Read the model definition and answer for the solid it produces. Units are mm, in the model's axes. A direction names the side the tool comes from. Coordinates: 2 decimals unless noted, no trailing zeros. Loops run counter-clockwise (first coordinate to the right, second up) from the corner with the lowest first, then second, coordinate; pieces in that order, holes last. Notation, with made-up numbers: (67, 78.25) -> (84, 78.25) arc R20 cw to (84, 116.25) -> close; hole circle Ø3 at (81, 89.25). An arc over 180 degrees is marked (long way). Answer as a JSON object with one key per item and string values. Group by question number.
1) Section C-C, the plane z = 2.05 is taken. Give the vertices of the cut face in (x, y), plus the area to 3 significant figures.
2) Which of the six approach directions +Z, -Z, +X, -X, +Y, -Y give full straight-line access (tool end or side, diameter ignored) to faces 1 (the face through (11, 0, 2)), 2 (the face through (-4.5, 0, 2)), 3 (the face through (3, -6, 2)), 4 (the face through (0, 0, 0)), 5 (the face through (3, 6, 2))?
3) Consider probe 1 along Y at (x, z) = (-1.5, 2.55); probe 2 along Z at (x, y) = (-6.25, 4); probe 3 along X at (y, z) = (1, 2.4). Determine where each line is inside the solid, lowest interval first. Write a range as [from, to].
4) Section A-A, the plane x = -4 is taken. Give the vertices of the cut face in (y, z).
5) Section B-B, the plane y = -3 is taken. Give the vertices of the cut face in (x, z), plus the area to 4 significant figures.
6) Flat-ended cylindrical pins translate along their axes: P1, Ø3, axis at x = 1.5, y = 6, coming from the -Z side; P2, Ø0.8, axis at y = -0.5, z = 2.5, coming from the -X side; P3, Ø1.6, axis at y = 0.5, z = 2.5, coming from the +X side. Find the tip coordinate at first contact, or state that the pin passes through.
from build123d import *

# Parameters (mm, degrees)
F0_W     = 24
F0_H     = 1.6
F1_DEPTH = 8
F2_W     = 15.5
F2_H     = 12
F3_DEPTH = 1.5


with BuildPart() as f1:
    # F0 (on Front) → F1 (new body, symmetric)
    with BuildSketch(Plane.XZ):
        with Locations((0, 0.8)):
            Rectangle(F0_W, F0_H)
    extrude(amount=F1_DEPTH, both=True)

    # F2 (on face) → F3 (join)
    with BuildSketch(Plane.XY.offset(1.6)):
        with Locations((3.25, 0)):
            Rectangle(F2_W, F2_H)
    extrude(amount=F3_DEPTH)


solid = f1.part
Determined:
{
 "1": {"outline": "(-4.5, -6) -> (11, -6) -> (11, 6) -> (-4.5, 6) -> close", "area": "186 mm²"},
 "2": {"face 1": "+Z, +X, +Y, -Y", "face 2": "+Z, -X, +Y, -Y", "face 3": "+Z, +X, -X, -Y", "face 4": "-Z, +X, -X, +Y, -Y", "face 5": "+Z, +X, -X, +Y"},
 "3": {"probe 1": "[-6, 6]", "probe 2": "[0, 1.6]", "probe 3": "[-4.5, 11]"},
 "4": {"outline": "(-8, 0) -> (8, 0) -> (8, 1.6) -> (6, 1.6) -> (6, 3.1) -> (-6, 3.1) -> (-6, 1.6) -> (-8, 1.6) -> close"},
 "5": {"outline": "(-12, 0) -> (12, 0) -> (12, 1.6) -> (11, 1.6) -> (11, 3.1) -> (-4.5, 3.1) -> (-4.5, 1.6) -> (-12, 1.6) -> close", "area": "61.65 mm²"},
 "6": {"P1": "z = 0", "P2": "x = -4.5", "P3": "x = 11"}
}
